from build123d import *

# Parameters (mm, degrees)
SKETCH1_W           = 45
SKETCH1_H           = 50
BOSS_EXTRUDE1_DEPTH = 45
SKETCH2_R           = 5.2
CUT_EXTRUDE1_DEPTH  = 45
SKETCH9_R           = 5.15
CUT_EXTRUDE6_DEPTH  = 2
SKETCH10_R          = 5.15
CUT_EXTRUDE7_DEPTH  = 2
SKETCH12_R          = 18.75
CUT_EXTRUDE8_DEPTH  = 50
SKETCH13_W          = 45
SKETCH13_H          = 6.66747138
CUT_EXTRUDE9_DEPTH  = 46
SKETCH14_W          = 45
SKETCH14_H          = 6.66747138
BOSS_EXTRUDE2_DEPTH = 45
SKETCH15_R          = 18.375
CUT_EXTRUDE10_DEPTH = 45
FILLET1_R           = 15
SKETCH16_R          = 18.75
BOSS_EXTRUDE3_DEPTH = 2
SKETCH18_R          = 18.75
CUT_EXTRUDE11_DEPTH = 43
SKETCH19_R          = 6.3
CUT_EXTRUDE12_DEPTH = 43
SKETCH20_R          = 1.7
CUT_EXTRUDE13_DEPTH = 43
SKETCH21_R          = 20
SKETCH21_R_2        = 18.75
BOSS_EXTRUDE4_DEPTH = 7
SKETCH22_R          = 18.75
SKETCH22_R_2        = 1.7
SKETCH22_R_3        = 6.3
BOSS_EXTRUDE5_DEPTH = 7
SKETCH23_R          = 18.75
SKETCH23_R_2        = 1.7
SKETCH23_R_3        = 6.3
CUT_EXTRUDE14_DEPTH = 7
SKETCH24_R          = 1.7
CUT_EXTRUDE15_DEPTH = 5
BOSS_EXTRUDE6_DEPTH = 2
SKETCH26_R          = 20
SKETCH26_R_2        = 6.3
SKETCH26_R_3        = 1.7
BOSS_EXTRUDE7_DEPTH = 10
SKETCH27_R          = 20
CUT_EXTRUDE16_DEPTH = 7


with BuildPart() as part:
    # Sketch1 → Boss-Extrude1 (new body)
    with BuildSketch(Plane.XY):
        with Locations((8.236607143, -2.901785714)):
            Rectangle(SKETCH1_W, SKETCH1_H)
    extrude(amount=BOSS_EXTRUDE1_DEPTH)

    # Sketch2 → Cut-Extrude1 (cut)
    with BuildSketch(Plane.XY.offset(45)):
        with Locations((-4.163392857, -24.901785714)):
            Circle(SKETCH2_R)
        with Locations((20.636607143, -24.901785714)):
            Circle(SKETCH2_R)
    extrude(amount=-CUT_EXTRUDE1_DEPTH, mode=Mode.SUBTRACT)

    # Sketch9 → Cut-Extrude6 (cut)
    with BuildSketch(Plane.XY.offset(45)):
        with Locations((8.236607143, -2.401785714)):
            Circle(SKETCH9_R)
    extrude(amount=-CUT_EXTRUDE6_DEPTH, mode=Mode.SUBTRACT)

    # Sketch10 → Cut-Extrude7 (cut)
    with BuildSketch(Plane(origin=(0, 0, 0), x_dir=(-1, 0, 0), z_dir=(0, 0, -1))):
        with Locations((-8.236607143, -2.401785714)):
            Circle(SKETCH10_R)
    extrude(amount=-CUT_EXTRUDE7_DEPTH, mode=Mode.SUBTRACT)

    # Sketch12 → Cut-Extrude8 (cut)
    with BuildSketch(Plane.ZY.offset(14.263392857)):
        with Locations((22.5, 1.098214286)):
            Circle(SKETCH12_R)
    extrude(amount=-CUT_EXTRUDE8_DEPTH, mode=Mode.SUBTRACT)

    # Sketch13 → Cut-Extrude9 (cut)
    with BuildSketch(Plane.ZY.offset(14.263392857)):
        with Locations((22.5, 18.764478596)):
            Rectangle(SKETCH13_W, SKETCH13_H)
    extrude(amount=-CUT_EXTRUDE9_DEPTH, mode=Mode.SUBTRACT)

    # Sketch14 → Boss-Extrude2 (add)
    with BuildSketch(Plane.ZY.offset(14.263392857)):
        with Locations((22.5, 18.764478596)):
            Rectangle(SKETCH14_W, SKETCH14_H)
    extrude(amount=-BOSS_EXTRUDE2_DEPTH)

    # Sketch15 → Cut-Extrude10 (cut)
    with BuildSketch(Plane.ZY.offset(14.263392857)):
        with Locations((22.5, 1.098214286)):
            Circle(SKETCH15_R)
    extrude(amount=-CUT_EXTRUDE10_DEPTH, mode=Mode.SUBTRACT)

    # Fillet1
    fillet1_edges = [part.edges().sort_by_distance(p)[0] for p in [
        (8.236607143, 22.098214286, 0),
        (8.236607143, 22.098214286, 45),
    ]]
    fillet(fillet1_edges, radius=FILLET1_R)

    # Sketch16 → Boss-Extrude3 (add)
    with BuildSketch(Plane(origin=(30.736607143, 0, 0), x_dir=(0, 0, -1), z_dir=(1, 0, 0))):
        with Locations((-22.5, 1.098214286)):
            Circle(SKETCH16_R)
    extrude(amount=-BOSS_EXTRUDE3_DEPTH)

    # Sketch18 → Cut-Extrude11 (cut)
    with BuildSketch(Plane.ZY.offset(14.263392857)):
        with Locations((22.5, 1.098214286)):
            Circle(SKETCH18_R)
    extrude(amount=-CUT_EXTRUDE11_DEPTH, mode=Mode.SUBTRACT)

    # Sketch19 → Cut-Extrude12 (cut)
    with BuildSketch(Plane(origin=(30.736607143, 0, 0), x_dir=(0, 0, -1), z_dir=(1, 0, 0))):
        with Locations((-22.5, 8.848214286)):
            Circle(SKETCH19_R)
    extrude(amount=-CUT_EXTRUDE12_DEPTH, mode=Mode.SUBTRACT)

    # Sketch20 → Cut-Extrude13 (cut)
    with BuildSketch(Plane(origin=(30.736607143, 0, 0), x_dir=(0, 0, -1), z_dir=(1, 0, 0))):
        with Locations((-6.05, 1.098214286)):
            Circle(SKETCH20_R)
    extrude(amount=-CUT_EXTRUDE13_DEPTH, mode=Mode.SUBTRACT)

    # Sketch21 → Boss-Extrude4 (add)
    with BuildSketch(Plane(origin=(30.736607143, 0, 0), x_dir=(0, 0, -1), z_dir=(1, 0, 0))):
        with Locations((-22.5, 1.098214286)):
            Circle(SKETCH21_R)
        with Locations((-22.5, 1.098214286)):
            Circle(SKETCH21_R_2, mode=Mode.SUBTRACT)
    extrude(amount=BOSS_EXTRUDE4_DEPTH)

    # Sketch22 → Boss-Extrude5 (add)
    with BuildSketch(Plane(origin=(30.736607143, 0, 0), x_dir=(0, 0, -1), z_dir=(1, 0, 0))):
        with Locations((-22.5, 1.098214286)):
            Circle(SKETCH22_R)
        with Locations((-6.05, 1.098214286)):
            Circle(SKETCH22_R_2, mode=Mode.SUBTRACT)
        with Locations((-22.5, 8.848214286)):
            Circle(SKETCH22_R_3, mode=Mode.SUBTRACT)
    extrude(amount=BOSS_EXTRUDE5_DEPTH)

    # Sketch23 → Cut-Extrude14 (cut)
    with BuildSketch(Plane.ZY.offset(-28.736607143)):
        with Locations((22.5, 1.098214286)):
            Circle(SKETCH23_R)
        with Locations((6.05, 1.098214286)):
            Circle(SKETCH23_R_2, mode=Mode.SUBTRACT)
        with Locations((22.5, 8.848214286)):
            Circle(SKETCH23_R_3, mode=Mode.SUBTRACT)
    extrude(amount=-CUT_EXTRUDE14_DEPTH, mode=Mode.SUBTRACT)

    # Sketch24 → Cut-Extrude15 (cut)
    with BuildSketch(Plane(origin=(37.736607143, 0, 0), x_dir=(0, 0, -1), z_dir=(1, 0, 0))):
        with Locations((-7.25882025, 1.098214286)):
            Circle(SKETCH24_R)
    extrude(amount=-CUT_EXTRUDE15_DEPTH, mode=Mode.SUBTRACT)

    # Sketch25 → Boss-Extrude6 (add)
    with BuildSketch(Plane(origin=(37.736607143, 0, 0), x_dir=(0, 0, -1), z_dir=(1, 0, 0))):
        with BuildLine():
            ThreePointArc((-6.654410125, 2.687141094), (-5.859267248, 2.063227961), (-5.55882025, 1.098214286))
            ThreePointArc((-5.55882025, 1.098214286), (-5.859267248, 0.13320061), (-6.654410125, -0.490712522))
            ThreePointArc((-6.654410125, -0.490712522), (-4.35, 1.098214286), (-6.654410125, 2.687141094))
        make_face()
    extrude(amount=-BOSS_EXTRUDE6_DEPTH)

    # Sketch26 → Boss-Extrude7 (add)
    with BuildSketch(Plane(origin=(37.736607143, 0, 0), x_dir=(0, 0, -1), z_dir=(1, 0, 0))):
        with Locations((-22.5, 1.098214286)):
            Circle(SKETCH26_R)
        with Locations((-22.5, 8.848214286)):
            Circle(SKETCH26_R_2, mode=Mode.SUBTRACT)
        with Locations((-7.25882025, 1.098214286)):
            Circle(SKETCH26_R_3, mode=Mode.SUBTRACT)
    extrude(amount=-BOSS_EXTRUDE7_DEPTH)

    # Sketch27 → Cut-Extrude16 (cut)
    with BuildSketch(Plane(origin=(37.736607143, 0, 0), x_dir=(0, 0, -1), z_dir=(1, 0, 0))):
        with Locations((-22.5, 1.098214286)):
            Circle(SKETCH27_R)
    extrude(amount=-CUT_EXTRUDE16_DEPTH, mode=Mode.SUBTRACT)


solid = part.part
The listing builds one solid part. Answer for the finished solid, in the listing's coordinates (mm). A direction names the side the tool comes from. Coordinates: 2 decimals unless noted, no trailing zeros. Order: outer loops, then holes, each group sorted by start corner. A loop starts at its lowest first (then second) coordinate and runs counter-clockwise, first axis right, second up. Notation, with made-up numbers: (21, -32.5) -> (42, -32.5) arc R36 ccw to (42, 1.5) -> close; hole circle Ø2 at (72, -22.5). An arc over 180 degrees is marked (long way). Answer in a Markdown table with one row per item. Add a question column.
Item 1: Find section C-C (z = 39.5). Write down the section's boundary in (x, y), then the cut area to 3 significant figures.
Item 2: Find the intervals of material crossed by L1, parallel to Z at x = -12, y = 0.5; L2, parallel to Y at x = 16, z = 22.5; L3, parallel to X at y = -23, z = 8.5, in increasing order. Write a range as from..to.
Item 3: Determine the mould class of faces 4 (the face through (30.737, -3, 23)), 5 (the face through (27.737, 1, 23)), 6 (the face through (8, -2, 43)), 7 (the face through (6, 10, 39)) for opening direction Z: +Z half, -Z half, draft (parallel to the pull), parting line (faces both ways), or undercut.
Item 4: Find section D-D (y = -4.5). Write down the section's boundary in (x, z), then the cut area to 3 significant figures.
Item 5: Each of these flat-tipped pins is pushed along its axis until it touches: P1, Ø1, axis at x = 16.5, y = 10, coming from the +Z side; P2, Ø12, axis at x = 8.24, y = -2.4, coming from the +Z side; P3, Ø6, axis at x = -9.5, z = 40, coming from the +Y side; P4, Ø5, axis at x = 7, y = -0.5, coming from the +Z side. Where does it stop, or does it pass through?
Item 6: Which of the six approach directions +Z, -Z, +X, -X, +Y, -Y give full straight-line access (tool end or side, diameter ignored) to faces 1 (the face through (8, 22.098, 22)), 2 (the face through (4.44, 1.08, 44.01)), 3 (the face through (8, -2, 2))?
Item 7: Find section A-A (z = 22.5). Write down the section's boundary in (x, y), then the cut area to 3 significant figures.
Item 8: Find section B-B (x = 12.5). Write down the section's boundary in (y, z).
Result set:
| question | item | result |
|---|---|---|
| 1 | outline | (-14.26, -27.9) -> (-8.41, -27.9) arc R5.2 cw (long way) to (0.08, -27.9) -> (16.39, -27.9) arc R5.2 cw (long way) to (24.88, -27.9) -> (30.74, -27.9) -> (30.74, 18.71) -> (-14.26, 18.71) -> (-14.26, 9.01) -> (27.74, 9.01) -> (27.74, -6.81) -> (-14.26, -6.81) -> close |
| 1 | area | 1,290 mm² |
| 2 | L1 | z = 0..3.76, 41.24..45 |
| 2 | L2 | y = -27.9..-27.26, -22.55..-17.65, 19.85..22.1 |
| 2 | L3 | x = -14.26..-9, 0.68..15.8, 25.48..30.74 |
| 3 | face 4 | draft |
| 3 | face 5 | undercut |
| 3 | face 6 | +Z half |
| 3 | face 7 | undercut |
| 4 | outline | (-14.26, 0) -> (3.53, 0) -> (3.53, 2) -> (12.94, 2) -> (12.94, 0) -> (30.74, 0) -> (30.74, 45) -> (12.94, 45) -> (12.94, 43) -> (3.53, 43) -> (3.53, 45) -> (-14.26, 45) -> (-14.26, 40.39) -> (27.74, 40.39) -> (27.74, 4.61) -> (-14.26, 4.61) -> close |
| 4 | area | 484 mm² |
| 5 | P1 | stops at z = 44.81 |
| 5 | P2 | stops at z = 45 |
| 5 | P3 | stops at y = 20.36 |
| 5 | P4 | stops at z = 43 |
| 6 | face 1 | +Z, -Z, +X, -X, +Y |
| 6 | face 2 | +Z |
| 6 | face 3 | -Z |
| 7 | outline | (-14.26, -27.9) -> (-8.41, -27.9) arc R5.2 cw (long way) to (0.08, -27.9) -> (16.39, -27.9) arc R5.2 cw (long way) to (24.88, -27.9) -> (30.74, -27.9) -> (30.74, 2.55) -> (27.74, 2.55) -> (27.74, -17.65) -> (-14.26, -17.65) -> close; (-14.26, 19.85) -> (27.74, 19.85) -> (27.74, 15.15) -> (30.74, 15.15) -> (30.74, 22.1) -> (-14.26, 22.1) -> close |
| 7 | area | 494 mm² |
| 8 | outline | (-27.9, 0) -> (-5.29, 0) -> (-5.29, 2) -> (0.49, 2) -> (0.49, 0) -> (7.1, 0) arc R15 ccw to (22.1, 15) -> (22.1, 30) arc R15 ccw to (7.1, 45) -> (0.49, 45) -> (0.49, 43) -> (-5.29, 43) -> (-5.29, 45) -> (-27.9, 45) -> close; hole circle Ø37.5 at (1.1, 22.5) |
